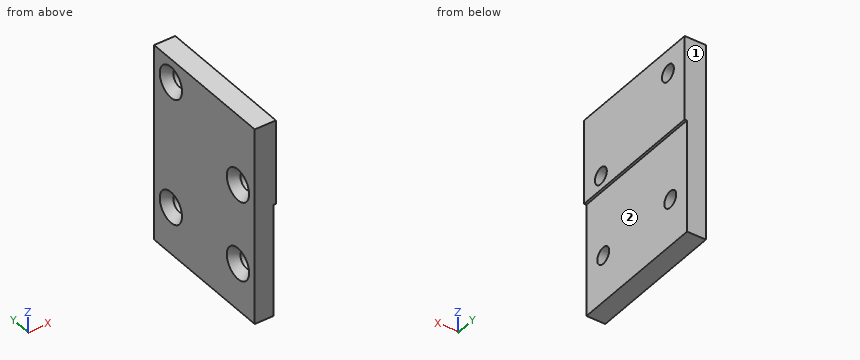
Autodesk Inventor part; units mm, degrees
ref_plane "YZ Plane" through (0, 0, 0) normal (1, 0, 0) x (0, 1, 0)
ref_plane "XZ Plane" through (0, 0, 0) normal (0, 1, 0) x (-1, 0, 0)
ref_plane "XY Plane" through (0, 0, 0) normal (0, 0, 1) x (1, 0, 0)
sketch "Sketch1" plane through (0, 0, 0) normal (1, 0, 0) x (0, 1, 0)
  line L0 (7.5884, 18.4529) -> (-30.5116, 18.4529)
  line L1 (-30.5116, 18.4529) -> (-30.5116, -34.8871)
  line L2 (-30.5116, -34.8871) -> (7.5884, -34.8871)
  line L3 (7.5884, -34.8871) -> (7.5884, 18.4529)
  point P0 (0, 0)
  dimension "d0" = 53.34
  dimension "d1" = 38.1
extrude "Extrusion1" add sketch "Sketch1" along normal blind 6.35
sketch "Sketch3" plane through (0, 7.5884, 18.4529) normal (0, 1, 0) x (1, 0, 0)
  line L0 (0, 22.86) -> (0.635, 22.86)
  line L1 (0.635, 22.86) -> (0.635, 53.34)
  line L2 (0.635, 53.34) -> (0, 53.34)
  line L3 (0, 53.34) -> (0, 22.86)
  line L4 (5.715, 53.34) -> (6.35, 53.34)
  line L5 (6.35, 53.34) -> (6.35, 22.86)
  line L6 (6.35, 22.86) -> (5.715, 22.86)
  line L7 (5.715, 22.86) -> (5.715, 53.34)
  line L8 (6.35, 53.34) -> (6.35, 0)
  line L9 (0, 53.34) -> (0, 0)
  line L10 (0, 53.34) -> (6.35, 53.34)
  point P0 (0, 18.4529)
  dimension "d19" = 30.48
  dimension "d20" = 30.48
  dimension "d21" = 0
  dimension "d22" = 0
  dimension "d23" = 0.635
  dimension "d24" = 0.635
  dimension "d25" = 0
extrude "Extrusion2" cut sketch "Sketch3" against normal blind 50.8
sketch "Sketch4" plane through (0, 7.5884, 18.4529) normal (0, 1, 0) x (1, 0, 0)
  line L0 (0.635, 34.7601) -> (-3.8704, 34.7601)
  line L1 (-3.8704, 34.7601) -> (-3.8704, -3.0853)
  line L2 (-3.8704, -3.0853) -> (0.635, -3.0853)
  line L3 (0.635, -3.0853) -> (0.635, 34.7601)
  line L4 (0.635, 53.34) -> (0.635, 22.86)
  point P0 (0, 18.4529)
  point P1 (0.635, 53.34)
  dimension "d28" = 0
extrude "Extrusion3" cut sketch "Sketch4" against normal blind 50.8
sketch "Sketch5" plane through (0.635, 7.5884, -34.8871) normal (-1, 0, 0) x (0, 0, 1)
  line L0 (53.34, 0) -> (53.34, -38.1)
  line L1 (0, 0) -> (53.34, 0)
  line L2 (0, -38.1) -> (0, 0)
  point P0 (34.8871, -7.5884)
  point P1 (46.99, -6.35)
  point P2 (34.29, -31.75)
  point P3 (53.34, -38.1)
  point P4 (12.7, -31.75)
  point P5 (12.7, -6.35)
  point P6 (52.07, -25.4)
  point P7 (5.08, 0)
  dimension "d31" = 6.35
  dimension "d32" = 6.35
  dimension "d33" = 31.75
  dimension "d34" = 19.05
  dimension "d35" = 31.75
  dimension "d36" = 12.7
  dimension "d37" = 12.7
  dimension "d38" = 6.35
hole "Hole2" at (0.635, 1.2384, 12.1029) at (0.635, -24.1616, -0.5971) at (0.635, -24.1616, -22.1871) at (0.635, 1.2384, -22.1871) direction (1, 0, 0) diameter 4.4958 end through all countersink diameter 8.4328 countersink angle 82
properties part number "GripperSidePlate"
Design review of the part built by this model. Coordinates are the model's own, in mm. Face numbers are marked on the shaded views. A direction names the side the tool comes from. Round coordinates to 2 decimals unless told otherwise and drop trailing zeros. Order: outer loops, then holes, each group sorted by start corner. A loop starts at its lowest first (then second) coordinate and runs counter-clockwise, first axis right, second up.
1) Consider section D-D (y = -23.5). Count the separate pieces of the cut face and the enclosed holes in it, plus the area to 3 significant figures.
The answers:
separate pieces: 3
enclosed holes: 0
area: 230 mm2
2) Consider section B-B (y = -12.5). State the section outline as (x, z) points (3 decimals).
The answers:
outline: (0.635, -34.887) - (5.715, -34.887) - (5.715, -4.407) - (6.35, -4.407) - (6.35, 18.453) - (0.635, 18.453) - close
3) Machinability: for the marked faces 1 and 2, which of the approach directions +Z, -Z, +X, -X, +Y, -Y give a long, thin tool a straight path to every point of the face, cutting with its end or side? Answer none if there is none.
The answers:
face 1: +Z, -Z, +X, -X, +Y
face 2: -Z, +X, +Y, -Y
4) Consider section A-A (x = 4.65). State the section outline as (y, z) points, plus the area to 3 significant figures.
The answers:
outline: (-30.51, -34.89) - (7.59, -34.89) - (7.59, 18.45) - (-30.51, 18.45) - close; hole circle Ø4.5 at (-24.16, -22.19); hole circle Ø4.5 at (-24.16, -0.6); hole circle Ø4.5 at (1.24, -22.19); hole circle Ø4.5 at (1.24, 12.1)
area: 1,970 mm2
5) Consider section C-C (z = -13). State the section outline as (x, y) points (3 decimals).
The answers:
outline: (0.635, -30.512) - (5.715, -30.512) - (5.715, 7.588) - (0.635, 7.588) - close
6) For L1, parallel to Z at x = 4.25, y = -24; L2, parallel to Y at x = 5.4, z = -24; L3, parallel to Z at x = 1.8, y = -25, list the stretches that pass through material, from the lowest coordinate up.
The answers:
L1: z = -34.89 to -24.43, -19.95 to -2.84, 1.64 to 18.45
L2: y = -30.51 to -25.49, -22.83 to -0.09, 2.57 to 7.59
L3: z = -34.89 to -25.28, -19.1 to -3.69, 2.49 to 18.45
